```python
from build123d import *

# Parameters (mm, degrees)
SKETCH_2_R          = 10.255
SKETCH_2_R_2        = 8.255
F_19MM_DEPTH        = 19
EXTRUDE_START       = -11
EXTRUDE_3_DEPTH     = 11
SKETCH_646_W        = 27.57
SKETCH_646_H        = 12
EXTRUDE_698_DEPTH   = 20
SKETCH_6_W          = 25.57
SKETCH_6_H          = 10
CUT_EXTRUDE_1_DEPTH = 15
FILLET_1_R          = 5
SKETCH_10_W         = 27.57
SKETCH_10_H         = 3
EXTRUDE_3_2_DEPTH   = 8


with BuildPart() as part:
    # 草圖2 → 19mm (new body)
    with BuildSketch(Plane(origin=(0, 0, 0), x_dir=(1, 0, 0), z_dir=(0, 1, 0))):
        Circle(SKETCH_2_R)
        Circle(SKETCH_2_R_2, mode=Mode.SUBTRACT)
    extrude(amount=F_19MM_DEPTH)

    # 草圖13 → Extrude 3 (add)
    with BuildSketch(Plane(origin=(0, 0, 0), x_dir=(1, 0, 0), z_dir=(0, 1, 0)).offset(EXTRUDE_START)):
        with BuildLine():
            ThreePointArc((-8.255, 0), (0, -8.255), (8.255, 0))
            Line((8.255, 0), (10.255, 0))
            ThreePointArc((10.255, 0), (0, -10.255), (-10.255, 0))
            Line((-10.255, 0), (-8.255, 0))
        make_face()
    extrude(amount=EXTRUDE_3_DEPTH)

    # Sketch 646 → Extrude 698 (add)
    with BuildSketch(Plane.XY):
        with Locations((0, -6)):
            Rectangle(SKETCH_646_W, SKETCH_646_H)
    extrude(amount=EXTRUDE_698_DEPTH)

    # 草圖6 → 除料-伸長1 (cut)
    with BuildSketch(Plane.XY.offset(20)):
        with Locations((0, -6)):
            Rectangle(SKETCH_6_W, SKETCH_6_H)
    extrude(amount=-CUT_EXTRUDE_1_DEPTH, mode=Mode.SUBTRACT)

    # 圓角1
    # the kernel refuses this fillet: 5 mm, written as the material it takes off along each edge
    with BuildSketch(Plane(origin=(-20.755, 0, 0), x_dir=(0, -1, 0), z_dir=(1, 0, 0))) as fillet_1_piece_1_section:
        with BuildLine():
            CenterArc((FILLET_1_R, -FILLET_1_R), FILLET_1_R, 90, 90)
            Line((0, -FILLET_1_R), (0, 0))
            Line((0, 0), (FILLET_1_R, 0))
        make_face()
    fillet_1_piece_1 = extrude(amount=41.51, mode=Mode.PRIVATE)
    fillet_1_piece_1 = fillet_1_piece_1 & Plane(origin=(0, -1.128045065, 0), x_dir=(1, 0, 0), z_dir=(0, -1, 0)) * Cylinder(8.255, 104, mode=Mode.PRIVATE)
    add(fillet_1_piece_1, mode=Mode.SUBTRACT)

    # 草圖10 → Extrude 3 2 (add)
    with BuildSketch(Plane.XZ.offset(12)):
        with Locations((0, 1.5)):
            Rectangle(SKETCH_10_W, SKETCH_10_H)
    extrude(amount=EXTRUDE_3_2_DEPTH)


solid = part.part
```
Could you check a few things on this model? Use its own coordinates, in mm. A direction names the side the tool comes from. Coordinates: 2 decimals unless noted, no trailing zeros. Write each loop counter-clockwise with the first axis right and the second up, starting at its lowest first coordinate (ties: lowest second). Pieces come first, ordered by that corner, then holes. Notation, with made-up numbers: (-40, 82.25) - (14, 82.25) arc R30 ccw to (14, 111.25) - close; hole circle Ø1 at (-27.75, -14). An arc over 180 degrees is marked (long way). Use a Markdown table: item, result.
Q1. Which directions (+Z, -Z, +X, -X, +Y, -Y) give clear straight access to the entire face, cutting with the end or side of a thin tool? Please do faces 5 (the flat face through (-12.785, -6, 13)), 6 (the flat face through (0, 0, 6)), 7 (the flat face through (0, -10, 0)).
Geometry check:
| item | result |
|---|---|
| face 5 | +Z |
| face 6 | +Y |
| face 7 | -Z, +X, -X, -Y |
Q2. Imagine slicing it at A-A (x = 0). List the corners of the cut face in (y, z) for me (3 decimals).
Geometry check:
| item | result |
|---|---|
| outline | (-20, 0) - (-5, 0) arc R5 ccw to (0, 5) - (0, 8.255) - (19, 8.255) - (19, 10.255) - (0, 10.255) - (0, 20) - (-1, 20) - (-1, 5) - (-11, 5) - (-11, 20) - (-12, 20) - (-12, 3) - (-20, 3) - close; (0, -10.255) - (19, -10.255) - (19, -8.255) - (0, -8.255) - close |
Q3. Imagine slicing it at B-B (z = 18.5). List the corners of the cut face in (x, y) for me (3 decimals).
Geometry check:
| item | result |
|---|---|
| outline | (-13.785, -12) - (13.785, -12) - (13.785, 0) - (-13.785, 0) - close; hole (-12.785, -11) - (12.785, -11) - (12.785, -1) - (-12.785, -1) - close |
Q4. I'm going to push flat-ended pins straight in: pin 1 Ø6 at (x, y) = (-3.5, 5) entering from -Z; pin 2 Ø11.5 at (x, z) = (-4.5, -7.5) entering from -Y; pin 3 Ø12 at (x, z) = (-8.5, 16.5) entering from +Y; pin 4 Ø1 at (y, z) = (-13, 5) entering from +X. Where does each tip first touch, or does it pass through?
Geometry check:
| item | result |
|---|---|
| pin 1 | stops at z = -10.24 |
| pin 2 | stops at y = 0 |
| pin 3 | stops at y = 0 |
| pin 4 | passes through |
Q5. Please list where these lines run through material, in increasing order: L1, parallel to Y at x = -7.25, z = 12; L2, parallel to Z at x = 0, y = 9.5 (3 decimals).
Geometry check:
| item | result |
|---|---|
| L1 | y = -12 to -11, -1 to 0 |
| L2 | z = -10.255 to -8.255, 8.255 to 10.255 |
Q6. Thinking about a two-plate mould opening in X: for faces 1 (the flat face through (0, -6, 5)), 2 (the flat face through (-13.785, -5, 10)), 3 (the flat face through (0, -12, 11)), 4 (the cylindrical face through (-8.14, 9.37, 6.24)), which applies, +X half, -X half, draft (parallel to the pull), parting line (faces both ways), or undercut?
Geometry check:
| item | result |
|---|---|
| face 1 | undercut |
| face 2 | -X half |
| face 3 | draft |
| face 4 | parting line |
Q7. Imagine slicing it at D-D (y = 16). List the corners of the cut face in (x, z) for me (3 decimals).
Geometry check:
| item | result |
|---|---|
| outline | circle Ø20.51 at (0, 0); hole circle Ø16.51 at (0, 0) |
Q8. Imagine slicing it at C-C (z = -7). List the corners of the cut face in (x, y) for me.
Geometry check:
| item | result |
|---|---|
| outline | (-7.49, 0) - (-4.38, 0) - (-4.38, 19) - (-7.49, 19) - close; (4.38, 0) - (7.49, 0) - (7.49, 19) - (4.38, 19) - close |
